Drawing for the job (mm, zero at the part's lowest x, y, z). Coordinates: 2 decimals unless noted, no trailing zeros. Order: outer loops, then holes, each group sorted by start corner. A loop starts at its lowest first (then second) coordinate and runs counter-clockwise, first axis right, second up.
1) Cut at B-B (y = 7.25). List the corners of the cut face in (x, z), and give its area (3 significant figures).
2) Wall check: L1, parallel to Z at x = 11, y = 6.75; L2, parallel to Z at x = 5, y = 2.5. Give the ranges that are in metal, low to high.
3) Pin check, flat tips, straight feed: pin 1 Ø1 at (x, y) = (9, 2) entering from +Z; pin 2 Ø0.8 at (x, z) = (16, 43.5) entering from +Y; pin 3 Ø0.8 at (x, z) = (16.5, 43.5) entering from -Y. Stop position of each tip, or through.
4) Cut at A-A (x = 7.5). List the corners of the cut face in (y, z).
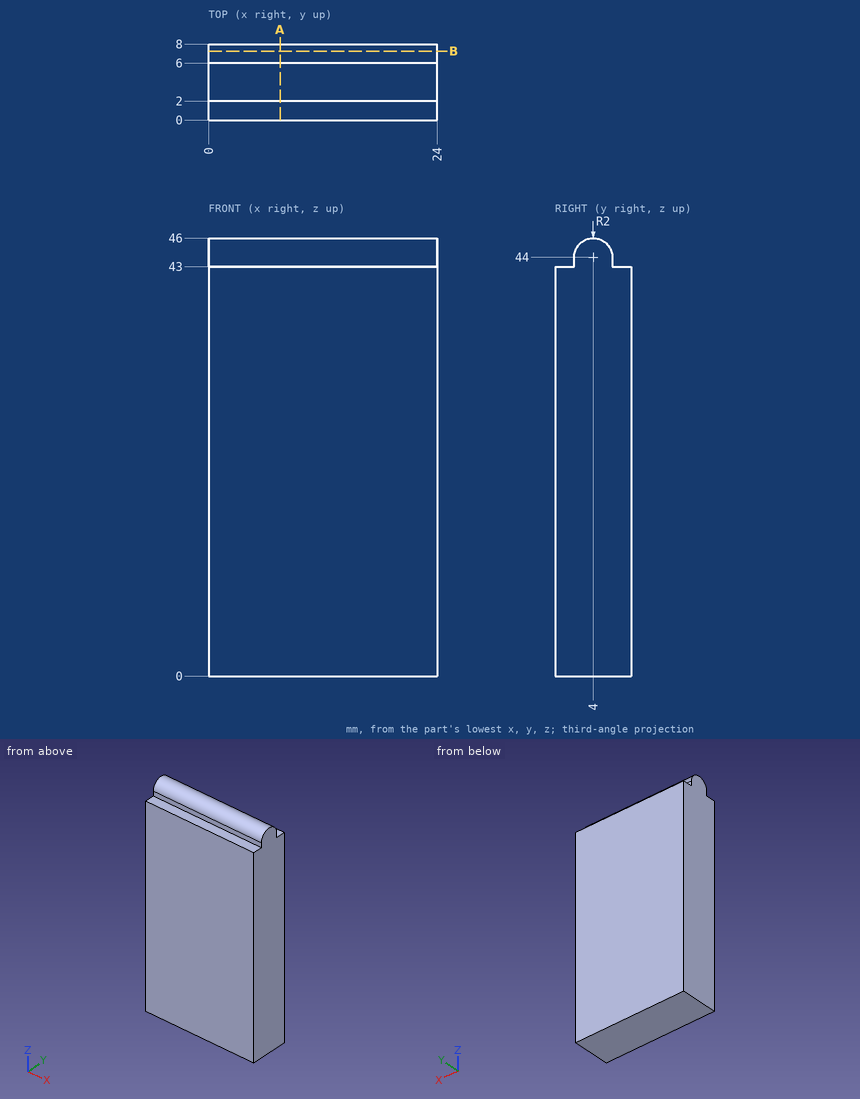
Geometry check:
1. outline: (0, 0) - (24, 0) - (24, 43) - (0, 43) - close
1. area: 1,030 mm2
2. L1: z = 0 to 43
2. L2: z = 0 to 45.32
3. pin 1: stops at z = 45.32
3. pin 2: stops at y = 6
3. pin 3: stops at y = 2
4. outline: (0, 0) - (8, 0) - (8, 43) - (6, 43) - (6, 44) arc R2 ccw to (2, 44) - (2, 43) - (0, 43) - close
